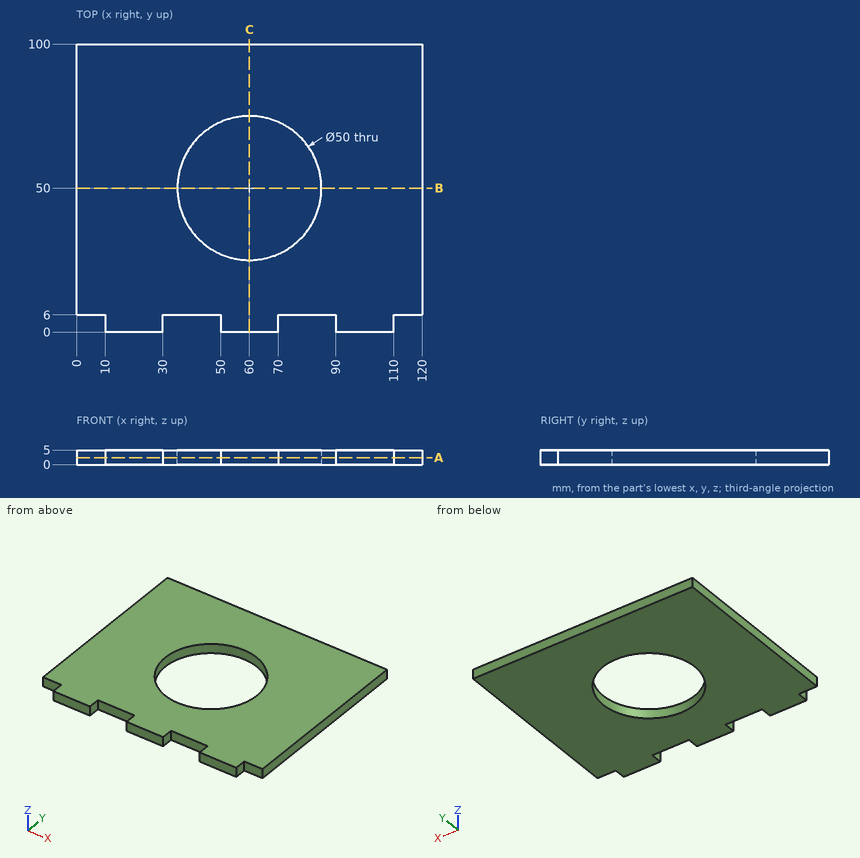
Design review of the part shown in the three views and the two pictorial views. Dimensions are in mm from the part's minimum x, y and z. Round coordinates to 2 decimals unless told otherwise and drop trailing zeros. Loops run counter-clockwise (first coordinate to the right, second up) from the corner with the lowest first, then second, coordinate; pieces in that order, holes last.
Q1. Add section C-C on x = 60. Write out the cut boundary in (y, z), plus the area to 3 significant figures.
Result sheet:
outline: (0, 0) - (25, 0) - (25, 5) - (0, 5) - close; (75, 0) - (100, 0) - (100, 5) - (75, 5) - close
area: 250 mm2
Q2. Insertion check: pin 1 Ø1.5 at (y, z) = (2, 3) entering from -X; pin 2 Ø2.5 at (x, z) = (5.5, 2.5) entering from -Y; pin 3 Ø1.5 at (y, z) = (2.5, 1.5) entering from +X. Each pin has a flat end and moves straight along its axis. Give the tip position at first contact, or say it passes through.
Result sheet:
pin 1: stops at x = 10
pin 2: stops at y = 6
pin 3: stops at x = 110
Q3. To check wall thickness, follow line 1 along Y through (x, z) = (59.5, 0.75) (3 decimals); line 2 along X through (y, z) = (65, 2.45); line 3 along X through (y, z) = (70.5, 4.6). State the ranges of each line that lie inside material, in increasing order.
Result sheet:
line 1: y = 0 to 25.005, 74.995 to 100
line 2: x = 0 to 40, 80 to 120
line 3: x = 0 to 45.69, 74.31 to 120
Q4. Add section B-B on y = 50. Write out the cut boundary in (x, z), plus the area to 3 significant figures.
Result sheet:
outline: (0, 0) - (35, 0) - (35, 5) - (0, 5) - close; (85, 0) - (120, 0) - (120, 5) - (85, 5) - close
area: 350 mm2
Q5. Add section A-A on z = 2.4. Write out the cut boundary in (x, y).
Result sheet:
outline: (0, 6) - (10, 6) - (10, 0) - (30, 0) - (30, 6) - (50, 6) - (50, 0) - (70, 0) - (70, 6) - (90, 6) - (90, 0) - (110, 0) - (110, 6) - (120, 6) - (120, 100) - (0, 100) - close; hole circle Ø50 at (60, 50)
